The listing builds one solid part. Answer for the finished solid, in the listing's coordinates (mm). A direction names the side the tool comes from. Coordinates: 2 decimals unless noted, no trailing zeros. Write each loop counter-clockwise with the first axis right and the second up, starting at its lowest first coordinate (ties: lowest second). Pieces come first, ordered by that corner, then holes.
```python
from build123d import *
from build123d.topology import SkipClean

# Parameters (mm, degrees)
SKETCH2_R           = 50
BOSS_EXTRUDE1_DEPTH = 100
CUT_EXTRUDE1_START  = -16.5
SKETCH3_R           = 50
SKETCH3_R_2         = 12.5
CUT_EXTRUDE1_DEPTH  = 16.5
CHAMFER2_SIZE       = 0.5
CHAMFER3_SIZE       = 3
CHAMFER3_SIZE_2     = 3.300188603


# Read off the part's stored shape, not the designer's step: Mirror1
with BuildPart() as part:
    # Sketch2 → Boss-Extrude1 (new body)
    with BuildSketch(Plane.YZ):
        with Locations(Location((0, 0, 0), (0, 0, 270))):
            Circle(SKETCH2_R)
    extrude(amount=BOSS_EXTRUDE1_DEPTH)

    # Sketch3 → Cut-Extrude1 (cut)
    with BuildSketch(Plane.YZ.offset(100).offset(CUT_EXTRUDE1_START)):
        with Locations(Location((0, 0, 0), (0, 0, 270))):
            Circle(SKETCH3_R)
        with Locations(Location((0, 0, 0), (0, 0, 270))):
            Circle(SKETCH3_R_2, mode=Mode.SUBTRACT)
    extrude(amount=CUT_EXTRUDE1_DEPTH, mode=Mode.SUBTRACT)

    # Chamfer2
    chamfer2_edges = [part.edges().sort_by_distance(p)[0] for p in [
        (100, 0, 12.5),
    ]]
    chamfer(chamfer2_edges, length=CHAMFER2_SIZE)

    # Sketch4 → Cut-Revolve2 (revolve, cut)
    with BuildSketch(Plane(origin=(0, 0, 0), x_dir=(-1, 0, 0), z_dir=(0, 1, 0))):
        Polygon((-83.5, 12.5), (-80.219175118, 50), (-83.5, 50), align=None)
    revolve(axis=Axis((0, 0, 0), (1, 0, 0)), mode=Mode.SUBTRACT)

    # Chamfer3
    # the kernel refuses this chamfer: 3.300188603, 3 mm, written as the material it takes off along each edge
    with BuildSketch(Plane(origin=(80.219175118, 0, 0), x_dir=(0, 0, 1), z_dir=(0, 1, 0))) as chamfer3_piece_1:
        Polygon((50 - CHAMFER3_SIZE * 0.996194698092, CHAMFER3_SIZE * 0.0871557427477), (50, -CHAMFER3_SIZE_2), (50, 0), align=None)
    revolve(axis=Axis((80.219175118, 0, 0), (1, 0, 0)), revolution_arc=180, mode=Mode.SUBTRACT)
    with BuildSketch(Plane(origin=(80.219175118, 0, 0), x_dir=(0, 0, -1), z_dir=(0, -1, 0))) as chamfer3_piece_2:
        Polygon((50 - CHAMFER3_SIZE * 0.996194698092, CHAMFER3_SIZE * 0.0871557427477), (50, -CHAMFER3_SIZE_2), (50, 0), align=None)
    revolve(axis=Axis((80.219175118, 0, 0), (1, 0, 0)), revolution_arc=180, mode=Mode.SUBTRACT)

    # Sketch7 → M10 Tapped Hole1 (revolve, cut)
    with BuildSketch(Plane(origin=(100, 0, 0), x_dir=(0, 0, -1), z_dir=(0, 1, 0))):
        Polygon((0, 0), (0, 59), (4.25, 56.446342369), (4.25, 50), (5, 50), (5, 0.025), (5.025, 0), align=None)
    revolve(axis=Axis((106.35, 0, 0), (-1, 0, 0)), mode=Mode.SUBTRACT)

    # Mirror1 outline → Mirror1 (revolve)
    with SkipClean():  # the faces are left unmerged after this step: merging them gives an invalid solid
        with BuildSketch(Plane.YX):
            Polygon((50, 0), (0, 0), (0, -41), (4.25, -43.553657631), (4.25, -50), (5, -50), (5, -99.975), (5.025, -100), (12, -100), (12.5, -99.5), (12.5, -83.5), (46.712369611, -80.506805507), (50, -77.219175118), align=None)
        revolve(axis=Axis((0, 0, 0), (1, 0, 0)))
    add(part.part.scale(1), mode=Mode.REPLACE)  # the faces are merged on a copy


solid = part.part
```
(1) Which of the six approach directions +Z, -Z, +X, -X, +Y, -Y give full straight-line access (tool end or side, diameter ignored) to faces 1 (the cylindrical face through (46.822, -3.584, -2.285)), 2 (the flat face through (100, 0.2, -5.2)), 3 (the cylindrical face through (-75.34, -1.08, -4.88))?
(2) Section B-B, the plane x = -30 is taken. Write down the section's boundary in (y, z), plus the area to 3 significant figures.
(3) Each of these flat-tipped pins is pushed along its axis until it touches: pin 1 (8 mm diameter, centred on x = -59.5, y = -19.5, fed in from -Z); pin 2 (5 mm diameter, centred on x = 39, z = -21.5, fed in from -Y); pin 3 (2 mm diameter, centred on y = -12, z = 21, fed in from +X) (3 decimals). Where does it stop, or does it pass through?
(4) Find the intervals of material crossed by probe 1 along Y at (x, z) = (67, 0); probe 2 along Z at (x, y) = (-46, 0); probe 3 along Z at (x, y) = (-16, 2), in increasing order.
(5) Section A-A, the plane x = -52 is taken. Write down the section's boundary in (y, z).
(6) For a pull along Y with two mould halves and no side action, classify faces 4 (the cylindrical face through (91.388, 3.755, -11.923)), 5 (the conical face through (-41.443, -0.16, -0.721)), 6 (the flat face through (-100, -5.2, 0.2)) as pulls with the +Y half, pulls with the -Y half, needs draft (parallel to the pull), parting line crosses it, or undercut.
Solution:
1. face 1: +X
1. face 2: +Z, -Z, +X, +Y, -Y
1. face 3: -X
2. outline: circle Ø100 at (0, 0)
2. area: 7,850 mm2
3. pin 1: stops at z = -47.54
3. pin 2: stops at y = -46.25
3. pin 3: stops at x = 82.565
4. probe 1: y = -50 to -5, 5 to 50
4. probe 2: z = -50 to -4.25, 4.25 to 50
4. probe 3: z = -49.96 to 49.96
5. outline: circle Ø100 at (0, 0); hole circle Ø10 at (0, 0)
6. face 4: parting line crosses it
6. face 5: undercut
6. face 6: needs draft
